```python
from build123d import *

# Parameters (mm, degrees)
F0_W     = 20
F0_H     = 20
F0_R     = 1.375
F0_R_2   = 5.5
F1_DEPTH = 3
F2_R     = 7.5
F2_R_2   = 5.5
F3_DEPTH = 4
F5_W     = 4.5
F5_H     = 2.413743116


with BuildPart() as f1:
    # F0 (on Top) → F1 (new body)
    with BuildSketch(Plane.XY):
        with Locations((10, 10)):
            Rectangle(F0_W, F0_H)
        with Locations((2.5, 2.5)):
            Circle(F0_R, mode=Mode.SUBTRACT)
        with Locations((17.5, 2.5)):
            Circle(F0_R, mode=Mode.SUBTRACT)
        with Locations((2.5, 17.5)):
            Circle(F0_R, mode=Mode.SUBTRACT)
        with Locations((10, 10)):
            Circle(F0_R_2, mode=Mode.SUBTRACT)
        with Locations((17.5, 17.5)):
            Circle(F0_R, mode=Mode.SUBTRACT)
    extrude(amount=F1_DEPTH)

    # F2 (on face) → F3 (join)
    with BuildSketch(Plane.XY.offset(3)):
        with Locations((10, 10)):
            Circle(F2_R)
        with Locations((10, 10)):
            Circle(F2_R_2, mode=Mode.SUBTRACT)
    extrude(amount=F3_DEPTH)

    # F5 (on offset) → F6 (revolve)
    with BuildSketch(Plane.XZ.offset(-10)):
        with Locations((15.25, 8.206871558)):
            Rectangle(F5_W, F5_H)
    revolve(axis=Axis((10, 10, 3.5), (0, 0, -1)))


solid = f1.part
```
Work out the finished part from the listing and answer in its coordinate system (mm). A direction names the side the tool comes from. Coordinates: 2 decimals unless noted, no trailing zeros. Write each loop counter-clockwise with the first axis right and the second up, starting at its lowest first coordinate (ties: lowest second). Pieces come first, ordered by that corner, then holes.
Q1. A cutting plane is placed at C-C, the plane x = 9.25. Give the vertices of the cut face in (y, z), then the cut area to 3 significant figures.
Q2. A cutting plane is placed at D-D, the plane z = 5. Give the vertices of the cut face in (x, y).
Q3. Each of these flat-tipped pins is pushed along its axis until it touches: pin 1 Ø4 at (x, y) = (11, 13) entering from -Z; pin 2 Ø7 at (x, y) = (10, 10) entering from +Z; pin 3 Ø5 at (x, z) = (8.5, 6) entering from -Y; pin 4 Ø3.5 at (x, y) = (17.5, 2.5) entering from +Z. Where does it stop, or does it pass through?
Q4. Determine the mould class of faces 4 (the face through (15.08, 7.89, 3.45)), 5 (the face through (8.37, 17.32, 6.25)), 6 (the face through (10, 0, 1)) for opening direction Y: released by +Y, released by -Y, zero draft, split by the parting line, or undercut.
Q5. A cutting plane is placed at B-B, the plane x = 1.75. Give the vertices of the cut face in (y, z), then the cut area to 3 significant figures.
Q6. Which of the six approach directions +Z, -Z, +X, -X, +Y, -Y give full straight-line access (tool end or side, diameter ignored) to faces 1 (the face through (7.6, 12.4, 7)), 2 (the face through (14, 3, 3)), 3 (the face through (16.126, 2.56, 1.479))?
Q7. A cutting plane is placed at A-A, the plane y = 10. Give the vertices of the cut face in (x, z), then the cut area to 3 significant figures.
Q8. Find the intervals of material crossed by line 1 (Y direction, x = 2.5, z = 2) (3 decimals); line 2 (X direction, y = 10, z = 8.7); line 3 (Z direction, x = 17.5, y = 6.5), in increasing order.
Findings below:
1. outline: (0, 0) - (4.55, 0) - (4.55, 7) - (7.1, 7) - (7.1, 9.41) - (2.54, 9.41) - (2.54, 3) - (0, 3) - close; (12.9, 7) - (15.45, 7) - (15.45, 0) - (20, 0) - (20, 3) - (17.46, 3) - (17.46, 9.41) - (12.9, 9.41) - close
1. area: 65.4 mm2
2. outline: circle Ø15 at (10, 10); hole circle Ø11 at (10, 10)
3. pin 1: stops at z = 7
3. pin 2: stops at z = 9.41
3. pin 3: stops at y = 2.5
3. pin 4: stops at z = 3
4. face 4: undercut
4. face 5: split by the parting line
4. face 6: released by -Y
5. outline: (0, 0) - (1.35, 0) - (1.35, 3) - (0, 3) - close; (3.65, 0) - (16.35, 0) - (16.35, 3) - (3.65, 3) - close; (18.65, 0) - (20, 0) - (20, 3) - (18.65, 3) - close
5. area: 46.2 mm2
6. face 1: -Z
6. face 2: +Z
6. face 3: +Z, -Z
7. outline: (0, 0) - (4.5, 0) - (4.5, 7) - (7, 7) - (7, 9.41) - (2.5, 9.41) - (2.5, 3) - (0, 3) - close; (13, 7) - (15.5, 7) - (15.5, 0) - (20, 0) - (20, 3) - (17.5, 3) - (17.5, 9.41) - (13, 9.41) - close
7. area: 64.7 mm2
8. line 1: y = 0 to 1.125, 3.875 to 16.125, 18.875 to 20
8. line 2: x = 2.5 to 7, 13 to 17.5
8. line 3: z = 0 to 3
